Can you work these out from the model? Positions are in its coordinate system, mm. A direction names the side the tool comes from. Coordinates: 2 decimals unless noted, no trailing zeros. Loops run counter-clockwise (first coordinate to the right, second up) from the corner with the lowest first, then second, coordinate; pieces in that order, holes last. Notation, with made-up numbers: (82.5, -37) -> (120.5, -37) arc R20 cw to (120.5, -24) -> close; hole circle Ø8 at (-39.75, 12.5). An arc over 180 degrees is marked (long way). Put each result on its own line as item: value. Start each with the question number.
Item 1: For faces 4 (the flat face through (-33.185, 2, 2)), 5 (the flat face through (11.025, -5.787, 2.348)), 6 (the flat face through (-8, 5, 4.762)), which set-ups out of +Z, -Z, +X, -X, +Y, -Y let a thin tool reach every point of the face, with its end or its side?
Item 2: We'd pull the mould along Y, two halves only. Please class faces 1 (the cylindrical face through (22.839, -7.555, 2.348)), 2 (the flat face through (-38.1, -10, 2)), 3 (the flat face through (0, -0.076, 2)): pulls with the +Y half, pulls with the -Y half, needs draft (parallel to the pull), parting line crosses it, or undercut.
Item 3: If we section it at B-B on y = 3: Please give me the cut outline in (x, z), plus the area to 3 significant figures.
Item 4: If we section it at C-C on y = -12.7: Please give me the cut outline in (x, z), plus the area to 3 significant figures.
Item 5: Please list where these lines run through material, in increasing order: L1, parallel to X at y = 12.7, z = 1.6; L2, parallel to X at y = 8, z = 1.9; L3, parallel to X at y = -13, z = 2.8. Write a range as from..to.
Item 6: If we section it at A-A on x = 3: Please give me the cut outline in (y, z), plus the area to 3 significant figures.
Item 7: Will these pins go through, and if not, where does the flat tip stop? P1, Ø2.5, axis at y = -0.5, z = 3.5, coming from the +X side; P2, Ø2.5, axis at y = 0.5, z = 2, coming from the -X side; P3, Ø2.5, axis at x = 35.72, y = 12.7, coming from the -Z side; P4, Ø1, axis at x = 12, z = 1.5, coming from the -Y side.
Item 8: If we section it at D-D on z = 2.4: State how many separate pieces and enclosed holes the cut face has, plus the area to 3 significant figures.
```python
from build123d import *

# Parameters (mm, degrees)
SKETCH2_R           = 1.4732
SKETCH2_W           = 9.6774
SKETCH2_H           = 12.8524
BOSS_EXTRUDE1_DEPTH = 4.7625


with BuildPart() as part:
    # Sketch2 → Boss-Extrude1 (new body)
    with BuildSketch(Plane.XY):
        with BuildLine():
            Line((-38.1, -16.51), (-38.1, -3.175))
            Line((-38.1, -3.175), (-33.1851, -3.175))
            Line((-33.1851, -3.175), (-33.1851, 6.35))
            Line((-33.1851, 6.35), (-38.1, 6.35))
            Line((-38.1, 6.35), (-38.1, 16.51))
            ThreePointArc((-38.1, 16.51), (-37.356051224, 18.306051224), (-35.56, 19.05))
            Line((-35.56, 19.05), (35.56, 19.05))
            ThreePointArc((35.56, 19.05), (37.356051224, 18.306051224), (38.1, 16.51))
            Line((38.1, 16.51), (38.1, 6.35))
            Line((38.1, 6.35), (33.1851, 6.35))
            Line((33.1851, 6.35), (33.1851, -3.175))
            Line((33.1851, -3.175), (38.1, -3.175))
            Line((38.1, -3.175), (38.1, -16.51))
            ThreePointArc((38.1, -16.51), (36.527699334, -18.858437353), (33.757355906, -18.299434064))
            Line((33.757355906, -18.299434064), (23.740904814, -8.209039139))
            ThreePointArc((23.740904814, -8.209039139), (22.825089709, -7.548328204), (21.745183011, -7.218089243))
            Line((21.745183011, -7.218089243), (0, -4.31608303))
            Line((0, -4.31608303), (-21.745183011, -7.218089243))
            ThreePointArc((-21.745183011, -7.218089243), (-22.825089709, -7.548328204), (-23.740904814, -8.209039139))
            Line((-23.740904814, -8.209039139), (-33.757355906, -18.299434064))
            ThreePointArc((-33.757355906, -18.299434064), (-36.527699334, -18.858437353), (-38.1, -16.51))
        make_face()
        with Locations(Location((-35.71875, 12.7, 0), (0, 0, 180))):
            Circle(SKETCH2_R, mode=Mode.SUBTRACT)
        with Locations(Location((-35.71875, -12.7, 0), (0, 0, 180))):
            Circle(SKETCH2_R, mode=Mode.SUBTRACT)
        with Locations(Location((35.71875, -12.7, 0), (0, 0, 180))):
            Circle(SKETCH2_R, mode=Mode.SUBTRACT)
        with Locations(Location((35.71875, 12.7, 0), (0, 0, 180))):
            Circle(SKETCH2_R, mode=Mode.SUBTRACT)
        with Locations(Location((-10.16, 6.335014615, 0), (0, 0, 180))):
            Circle(SKETCH2_R, mode=Mode.SUBTRACT)
        with Locations(Location((10.16, 6.335014615, 0), (0, 0, 180))):
            Circle(SKETCH2_R, mode=Mode.SUBTRACT)
        with Locations((0, 6.35)):
            Rectangle(SKETCH2_W, SKETCH2_H, mode=Mode.SUBTRACT)
    extrude(amount=BOSS_EXTRUDE1_DEPTH)


solid = part.part
```
Solutions:
1. face 4: +Z, -Z, -X
1. face 5: +Z, -Z, -Y
1. face 6: +Z, +X, -X, +Y, -Y
2. face 1: pulls with the -Y half
2. face 2: needs draft
2. face 3: undercut
3. outline: (-33.19, 0) -> (-4.84, 0) -> (-4.84, 4.76) -> (-33.19, 4.76) -> close; (4.84, 0) -> (33.19, 0) -> (33.19, 4.76) -> (4.84, 4.76) -> close
3. area: 270 mm^2
4. outline: (-38.1, 0) -> (-37.19, 0) -> (-37.19, 4.76) -> (-38.1, 4.76) -> close; (-34.25, 0) -> (-28.2, 0) -> (-28.2, 4.76) -> (-34.25, 4.76) -> close; (28.2, 0) -> (34.25, 0) -> (34.25, 4.76) -> (28.2, 4.76) -> close; (37.19, 0) -> (38.1, 0) -> (38.1, 4.76) -> (37.19, 4.76) -> close
4. area: 66.2 mm^2
5. L1: -38.1..-37.19, -34.25..-4.84, 4.84..34.25, 37.19..38.1
5. L2: -38.1..-4.84, 4.84..38.1
5. L3: -38.1..-37.16, -34.28..-28.5, 28.5..34.28, 37.16..38.1
6. outline: (-4.72, 0) -> (-0.08, 0) -> (-0.08, 4.76) -> (-4.72, 4.76) -> close; (12.78, 0) -> (19.05, 0) -> (19.05, 4.76) -> (12.78, 4.76) -> close
6. area: 52.0 mm^2
7. P1: x = 33.19
7. P2: x = -33.19
7. P3: through
7. P4: y = -5.98
8. separate pieces: 1
8. enclosed holes: 7
8. area: 1,900 mm^2
